from build123d import *

# Parameters (mm, degrees)
SKETCH1_W           = 170
SKETCH1_H           = 280
BOSS_EXTRUDE1_DEPTH = 90
CUT_EXTRUDE1_DEPTH  = 90
CUT_EXTRUDE2_DEPTH  = 90
SKETCH4_W           = 20
SKETCH4_H           = 35
CUT_EXTRUDE3_DEPTH  = 299
CUT_EXTRUDE4_DEPTH  = 40
SKETCH6_R           = 9
CUT_EXTRUDE5_DEPTH  = 50
CUT_EXTRUDE6_DEPTH  = 35
SKETCH8_R           = 9
CUT_EXTRUDE7_DEPTH  = 35
CUT_EXTRUDE9_DEPTH  = 15
SKETCH10_R          = 20
BOSS_EXTRUDE2_DEPTH = 35
SKETCH11_R          = 9
CUT_EXTRUDE10_DEPTH = 35
SKETCH12_W          = 5
SKETCH12_H          = 20
SKETCH12_H_2        = 20.204959883
BOSS_EXTRUDE3_DEPTH = 25
CUT_EXTRUDE11_DEPTH = 35
CUT_EXTRUDE12_DEPTH = 10


with BuildPart() as part:
    # Sketch1 → Boss-Extrude1 (new body)
    with BuildSketch(Plane.XY):
        with Locations((85, 140)):
            Rectangle(SKETCH1_W, SKETCH1_H)
    extrude(amount=BOSS_EXTRUDE1_DEPTH)

    # Sketch2 → Cut-Extrude1 (cut)
    with BuildSketch(Plane.XY.offset(90)):
        with BuildLine():
            Line((0, 280), (0, 195))
            ThreePointArc((0, 195), (24.895923599, 255.104076401), (85, 280))
            Line((85, 280), (0, 280))
        make_face()
        with BuildLine():
            Line((170, 280), (85, 280))
            ThreePointArc((85, 280), (145.104076401, 255.104076401), (170, 195))
            Line((170, 195), (170, 280))
        make_face()
    extrude(amount=-CUT_EXTRUDE1_DEPTH, mode=Mode.SUBTRACT)

    # Sketch3 → Cut-Extrude2 (cut)
    with BuildSketch(Plane.XY.offset(90)):
        with BuildLine():
            Line((15, 0), (155, 0))
            ThreePointArc((155, 0), (85, 70), (15, 0))
        make_face()
    extrude(amount=-CUT_EXTRUDE2_DEPTH, mode=Mode.SUBTRACT)

    # Sketch4 → Cut-Extrude3 (cut)
    with BuildSketch(Plane(origin=(0, 0, 0), x_dir=(1, 0, 0), z_dir=(0, 1, 0))):
        with Locations((10, -72.5)):
            Rectangle(SKETCH4_W, SKETCH4_H)
        with Locations((160, -72.5)):
            Rectangle(SKETCH4_W, SKETCH4_H)
    extrude(amount=CUT_EXTRUDE3_DEPTH, mode=Mode.SUBTRACT)

    # Sketch5 → Cut-Extrude4 (cut)
    with BuildSketch(Plane(origin=(0, 0, 0), x_dir=(-1, 0, 0), z_dir=(0, 0, -1))):
        with BuildLine():
            Line((-20, 25.980762114), (-20, 195))
            ThreePointArc((-20, 195), (-85, 260), (-150, 195))
            Line((-150, 195), (-150, 25.980762114))
            ThreePointArc((-150, 25.980762114), (-85, 70), (-20, 25.980762114))
        make_face()
    extrude(amount=-CUT_EXTRUDE4_DEPTH, mode=Mode.SUBTRACT)

    # Sketch6 → Cut-Extrude5 (cut)
    with BuildSketch(Plane.XY.offset(90)):
        with Locations((85, 90)):
            Circle(SKETCH6_R)
    extrude(amount=-CUT_EXTRUDE5_DEPTH, mode=Mode.SUBTRACT)

    # Sketch7 → Cut-Extrude6 (cut)
    with BuildSketch(Plane.XY.offset(90)):
        with BuildLine():
            Line((20, 90), (20, 249.772255751))
            ThreePointArc((20, 249.772255751), (85, 280), (150, 249.772255751))
            Line((150, 249.772255751), (150, 90))
            ThreePointArc((150, 90), (85, 155), (20, 90))
        make_face()
    extrude(amount=-CUT_EXTRUDE6_DEPTH, mode=Mode.SUBTRACT)

    # Sketch8 → Cut-Extrude7 (cut)
    with BuildSketch(Plane.XY.offset(90)):
        with BuildLine():
            ThreePointArc((120, 90), (85, 125), (50, 90))
            Line((50, 90), (50, 60.621778265))
            ThreePointArc((50, 60.621778265), (85, 70), (120, 60.621778265))
            Line((120, 60.621778265), (120, 90))
        make_face()
        with Locations((85, 90)):
            Circle(SKETCH8_R, mode=Mode.SUBTRACT)
    extrude(amount=-CUT_EXTRUDE7_DEPTH, mode=Mode.SUBTRACT)

    # Sketch9 → Cut-Extrude9 (cut)
    with BuildSketch(Plane.XY.offset(80)):
        with BuildLine():
            Line((35, 90), (50, 90))
            ThreePointArc((50, 90), (85, 125), (120, 90))
            Line((120, 90), (135, 90))
            ThreePointArc((135, 90), (85, 140), (35, 90))
        make_face()
        with BuildLine():
            Line((50, 90), (35, 90))
            Line((35, 90), (35, 48.989794856))
            ThreePointArc((35, 48.989794856), (85, 70), (135, 48.989794856))
            Line((135, 48.989794856), (135, 90))
            Line((135, 90), (120, 90))
            ThreePointArc((120, 90), (85, 125), (50, 90))
        make_face()
    extrude(amount=-CUT_EXTRUDE9_DEPTH, mode=Mode.SUBTRACT)

    # Sketch10 → Boss-Extrude2 (add)
    with BuildSketch(Plane.XY.offset(55)):
        with Locations((85, 195)):
            Circle(SKETCH10_R)
    extrude(amount=BOSS_EXTRUDE2_DEPTH)

    # Sketch11 → Cut-Extrude10 (cut)
    with BuildSketch(Plane.XY.offset(90)):
        with Locations((85, 195)):
            Circle(SKETCH11_R)
    extrude(amount=-CUT_EXTRUDE10_DEPTH, mode=Mode.SUBTRACT)

    # Sketch12 → Boss-Extrude3 (add)
    with BuildSketch(Plane.XY.offset(55)):
        with Locations((85, 224.843134833)):
            Rectangle(SKETCH12_W, SKETCH12_H)
        with Locations((85, 165.054385226)):
            Rectangle(SKETCH12_W, SKETCH12_H_2)
    extrude(amount=BOSS_EXTRUDE3_DEPTH)

    # Sketch13 → Cut-Extrude11 (cut)
    with BuildSketch(Plane.XY.offset(55)):
        with BuildLine():
            ThreePointArc((3.759615954, 220), (42.697632957, 235.393046487), (56.277186767, 275))
            ThreePointArc((56.277186767, 275), (23.524588745, 253.700713889), (3.759615954, 220))
        make_face()
        with BuildLine():
            ThreePointArc((166.240384046, 220), (146.475411255, 253.700713889), (113.722813233, 275))
            ThreePointArc((113.722813233, 275), (127.302367043, 235.393046487), (166.240384046, 220))
        make_face()
    extrude(amount=-CUT_EXTRUDE11_DEPTH, mode=Mode.SUBTRACT)

    # Sketch14 → Cut-Extrude12 (cut)
    with BuildSketch(Plane(origin=(87.5, 0, 0), x_dir=(0, 0, -1), z_dir=(1, 0, 0))):
        Polygon((-80, 214.843134833), (-55, 234.843134833), (-80, 234.843134833), align=None)
    extrude(amount=-CUT_EXTRUDE12_DEPTH, mode=Mode.SUBTRACT)


solid = part.part
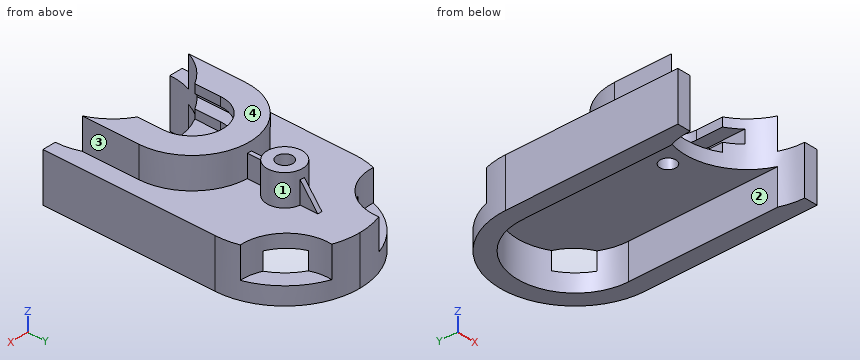
Geometry: final body of the model. Coordinates: model frame, mm. Face numbers are marked on the shaded views. A direction names the side the tool comes from. Give positions to 0.01 mm unless a question says otherwise; leave off trailing zeros. Write each loop counter-clockwise with the first axis right and the second up, starting at its lowest first coordinate (ties: lowest second). Pieces come first, ordered by that corner, then holes.
(1) Ray query, line 1 (Y direction, x = 86, z = 82); line 2 (X direction, y = 62.5, z = 61.5); line 3 (Y direction, x = 85, z = 46.75). Return the intervals inside material, ascending.
(2) First-contact query: P1, Ø17.5, axis at y = 72, z = 65.5, coming from the -X side; P2, Ø8, axis at x = 140, z = 79, coming from the -Y side; P3, Ø14.5, axis at x = 85.5, y = 195.5, coming from the +Z side. Flat tips, straight axial feed; report the tip coordinate or a pass-through.
(3) Cut plane B-B, the plane x = 40. Return loops of the section in (y, z).
(4) Cut plane A-A, the plane y = 163. Return loops of the section in (x, z), then the cut area to 4 significant figures.
(5) Cut plane C-C, the plane z = 36. Return loops of the section in (x, y), then the cut area to 3 significant figures.
(6) Access query for the marked faces 1, 2, 3 and 4. Directions: +Z, -Z, +X, -X, +Y, -Y. A direction counts if a zero-diameter tool reaches every point of the face in a straight line with its end or side. Return the directions, or none.
(7) Cut plane D-D, the plane z = 11.5. Return loops of the section in (x, y).
Values follow:
1. line 1: y = 124.99 to 154.99, 175.03 to 186.06, 203.94 to 214.97
1. line 2: x = 20 to 50, 120 to 150
1. line 3: y = 70 to 81, 99 to 280
2. P1: stops at x = 20
2. P2: stops at y = 37.67
2. P3: stops at z = 55
3. outline: (53.62, 40) - (232.77, 40) - (232.77, 55) - (136.9, 55) - (136.9, 90) - (53.62, 90) - (53.62, 80) - (111.79, 80) - (111.79, 65) - (53.62, 65) - close; (241.9, 0) - (267.11, 0) - (267.11, 20) - (241.9, 20) - close
4. outline: (0, 0) - (20, 0) - (20, 40) - (150, 40) - (150, 0) - (170, 0) - (170, 55) - (87.5, 55) - (87.5, 80) - (82.5, 80) - (82.5, 55) - (0, 55) - close
4. area: 4,275 mm2
5. outline: (0, 0) - (15, 0) arc R70 cw to (20, 25.98) - (20, 195) arc R65 cw to (26.97, 224.29) arc R50 cw to (3.76, 220) arc R85 ccw to (0, 195) - close; (53.06, 251.61) arc R65 cw to (116.94, 251.61) arc R50 cw to (113.72, 275) arc R85 ccw to (56.28, 275) arc R50 cw to start; (143.03, 224.29) arc R65 cw to (150, 195) - (150, 25.98) arc R70 cw to (155, 0) - (170, 0) - (170, 195) arc R85 ccw to (166.24, 220) arc R50 cw to start
5. area: 9,900 mm2
6. face 1: +Z
6. face 2: -Z, -Y
6. face 3: +Z, +X, +Y, -Y
6. face 4: +Z, +X, -X, +Y, -Y
7. outline: (0, 0) - (15, 0) arc R70 cw to (20, 25.98) - (20, 195) arc R65 cw to (150, 195) - (150, 25.98) arc R70 cw to (155, 0) - (170, 0) - (170, 195) arc R85 ccw to (0, 195) - close
